```python
from build123d import *

# Parameters (mm, degrees)
SKETCH2_W            = 75
SKETCH2_H            = 25
BOSS_EXTRUDE1_DEPTH  = 1.5
BOSS_EXTRUDE5_DEPTH  = 25
BOSS_EXTRUDE5_TAPER  = 1
SKETCH6_W            = 75
SKETCH6_H            = 0.75
BOSS_EXTRUDE6_DEPTH  = 2
BOSS_EXTRUDE7_REACH  = 85.38
BOSS_EXTRUDE8_DEPTH  = 0.436377
SKETCH10_W           = 0.281811688
SKETCH10_H           = 25
BOSS_EXTRUDE9_DEPTH  = 2
SKETCH13_W           = 4
SKETCH13_H           = 25
BOSS_EXTRUDE10_DEPTH = 6
SKETCH14_W           = 4
SKETCH14_H           = 25
BOSS_EXTRUDE11_DEPTH = 6
SKETCH15_R           = 1.75
CUT_EXTRUDE1_DEPTH   = 6
SKETCH16_W           = 0.3
SKETCH16_H           = 25
BOSS_EXTRUDE12_DEPTH = 0.8


with BuildPart() as part:
    # Sketch2 → Boss-Extrude1 (new body)
    with BuildSketch(Plane(origin=(0, 0, 0), x_dir=(1, 0, 0), z_dir=(0, 1, 0))):
        with Locations((37.5, 12.5)):
            Rectangle(SKETCH2_W, SKETCH2_H)
    extrude(amount=BOSS_EXTRUDE1_DEPTH)

    # Sketch4 → Boss-Extrude5 (add)
    with BuildSketch(Plane(origin=(0, 1.5, 0), x_dir=(1, 0, 0), z_dir=(0, 1, 0))):
        Polygon((24, 25), (0, 25), (0, 0), (1, 0), (1, 24), (24, 24), (24, 0), (26, 0), (26, 24), (49, 24), (49, 0), (51, 0), (51, 24), (74, 24), (74, 0), (75, 0), (75, 25), (51, 25), (49, 25), (26, 25), align=None)
    extrude(amount=BOSS_EXTRUDE5_DEPTH, taper=BOSS_EXTRUDE5_TAPER)

    # Sketch6 → Boss-Extrude6 (add)
    with BuildSketch(Plane.XY):
        with Locations((37.5, 1.125)):
            Rectangle(SKETCH6_W, SKETCH6_H)
    extrude(amount=BOSS_EXTRUDE6_DEPTH)

    # Boss-Extrude7: up to this face of the body (flat: up to its plane)
    boss_extrude7_end = Plane(part.part.faces().sort_by_distance((37.5, 1.5, -10.920265781))[0])
    # Sketch8 → Boss-Extrude7 (add, up to the picked face)
    with BuildSketch(Plane(origin=(0, 26.5, 0), x_dir=(1, 0, 0), z_dir=(0, 1, 0)), mode=Mode.PRIVATE) as boss_extrude7_sk1:
        Polygon((0, 25), (0, 0), (0.436376623, 0.436376623), (0.436376623, 24.563623377), (74.563623377, 24.563623377), (74.563623377, 0.436376623), (75, 0), (75, 25), align=None)
    boss_extrude7_tool1 = split(extrude(boss_extrude7_sk1.sketch, amount=-BOSS_EXTRUDE7_REACH, mode=Mode.PRIVATE), bisect_by=boss_extrude7_end, keep=Keep.BOTH, mode=Mode.PRIVATE)
    add(boss_extrude7_tool1.solids().sort_by(Axis((0.079057, 26.5, -12.5), (0, -1, 0)))[0])

    # Sketch9 → Boss-Extrude8 (add)
    with BuildSketch(Plane(origin=(0, 0, 0), x_dir=(-1, 0, 0), z_dir=(0, 0, -1))):
        Polygon((-75, 1.5), (-75, 26.5), (-74.563623377, 26.5), (-74.436376623, 26.5), (-74, 1.5), align=None)
        Polygon((-49, 1.5), (-51, 1.5), (-50.563623377, 26.5), (-49.436376623, 26.5), align=None)
        Polygon((-0.436376623, 26.5), (0, 26.5), (0, 1.5), (-1, 1.5), (-0.563623377, 26.5), align=None)
        Polygon((-24, 1.5), (-26, 1.5), (-25.563623377, 26.5), (-24.436376623, 26.5), align=None)
    extrude(amount=BOSS_EXTRUDE8_DEPTH)

    # Sketch10 → Boss-Extrude9 (add)
    with BuildSketch(Plane.XY):
        with Locations((0.140905844, 14)):
            Rectangle(SKETCH10_W, SKETCH10_H)
        with Locations((74.859094156, 14)):
            Rectangle(SKETCH10_W, SKETCH10_H)
    extrude(amount=BOSS_EXTRUDE9_DEPTH)

    # Sketch13 → Boss-Extrude10 (add)
    with BuildSketch(Plane.ZY):
        with Locations((-2, 14)):
            Rectangle(SKETCH13_W, SKETCH13_H)
    extrude(amount=BOSS_EXTRUDE10_DEPTH)

    # Sketch14 → Boss-Extrude11 (add)
    with BuildSketch(Plane(origin=(75, 0, 0), x_dir=(0, 0, -1), z_dir=(1, 0, 0))):
        with Locations((2, 14)):
            Rectangle(SKETCH14_W, SKETCH14_H)
    extrude(amount=BOSS_EXTRUDE11_DEPTH)

    # Sketch15 → Cut-Extrude1 (cut)
    with BuildSketch(Plane.XY):
        with Locations((-3, 24)):
            Circle(SKETCH15_R)
        with Locations((78, 24)):
            Circle(SKETCH15_R)
        with Locations((-3, 14)):
            Circle(SKETCH15_R)
        with Locations((-3, 4)):
            Circle(SKETCH15_R)
        with Locations((78, 14)):
            Circle(SKETCH15_R)
        with Locations((78, 4)):
            Circle(SKETCH15_R)
    extrude(amount=-CUT_EXTRUDE1_DEPTH, mode=Mode.SUBTRACT)

    # Sketch16 → Boss-Extrude12 (add)
    with BuildSketch(Plane.XY):
        with Locations((25, 14)):
            Rectangle(SKETCH16_W, SKETCH16_H)
        with Locations((50, 14)):
            Rectangle(SKETCH16_W, SKETCH16_H)
    extrude(amount=BOSS_EXTRUDE12_DEPTH)


solid = part.part
```
Can you work these out from the model? Positions are in its coordinate system, mm. A direction names the side the tool comes from. Coordinates: 2 decimals unless noted, no trailing zeros. Loops run counter-clockwise (first coordinate to the right, second up) from the corner with the lowest first, then second, coordinate; pieces in that order, holes last.
Item 1: Please list where these lines run through material, in increasing order: L1, parallel to Y at x = -3, z = -0.85; L2, parallel to X at y = 21, z = -20.75; L3, parallel to X at y = 3, z = -11.5.
Answers below:
L1: y = 1.5 to 2.25, 5.75 to 12.25, 15.75 to 22.25, 25.75 to 26.5
L2: x = 0 to 0.66, 24.34 to 25.66, 49.34 to 50.66, 74.34 to 75
L3: x = 0 to 0.97, 24.03 to 25.97, 49.03 to 50.97, 74.03 to 75
Item 2: I'm going to push flat-ended pins straight in: pin 1 (6 mm diameter, centred on y = 4.5, z = -19.5, fed in from -X); pin 2 (8 mm diameter, centred on x = 11.5, y = 15, fed in from +Z); pin 3 (8 mm diameter, centred on y = 18, z = -10.5, fed in from +X). Where does each tip first touch, or does it pass through?
Answers below:
pin 1: stops at x = 0
pin 2: stops at z = -24.17
pin 3: stops at x = 75
Item 3: Suppose I cut it at B-B (z = -3). State how many separate pieces and enclosed holes the cut face has, then the cut area to 3 significant figures.
Answers below:
separate pieces: 1
enclosed holes: 6
area: 472 mm2
Item 4: Which directions (+Z, -Z, +X, -X, +Y, -Y) give clear straight access to the entire face, cutting with the end or side of a thin tool? Please do faces 4 (the face through (-1, 14, 0)), 5 (the face through (37, 0.75, 1)), 6 (the face through (-3.228, 15.735, -1.972)), 7 (the face through (-3, 1.5, -2)), 8 (the face through (78, 1.5, -2)).
Answers below:
face 4: +Z, -X, +Y, -Y
face 5: +Z, +X, -X, -Y
face 6: +Z, -Z
face 7: +Z, -Z, -X, -Y
face 8: +Z, -Z, +X, -Y
Item 5: Suppose I cut it at A-A (x = -3). Please give me the cut outline in (y, z).
Answers below:
outline: (1.5, -4) - (2.25, -4) - (2.25, 0) - (1.5, 0) - close; (5.75, -4) - (12.25, -4) - (12.25, 0) - (5.75, 0) - close; (15.75, -4) - (22.25, -4) - (22.25, 0) - (15.75, 0) - close; (25.75, -4) - (26.5, -4) - (26.5, 0) - (25.75, 0) - close
Item 6: If we mould it in two halves opening along Y, with no side actions, what happens to faces 1 (the face through (37, 0, -13)), 2 (the face through (76, 14, 0)), 3 (the face through (-3.38, 2.29, -1.97))? For each: released by +Y, released by -Y, zero draft, split by the parting line, or undercut.
Answers below:
face 1: released by -Y
face 2: zero draft
face 3: undercut
